Autodesk Inventor part; units mm, degrees
ref_plane "YZ Plane" through (0, 0, 0) normal (1, 0, 0) x (0, 1, 0)
ref_plane "XZ Plane" through (0, 0, 0) normal (0, 1, 0) x (-1, 0, 0)
ref_plane "XY Plane" through (0, 0, 0) normal (0, 0, 1) x (1, 0, 0)
sketch "Sketch1" plane through (0, 0, 0) normal (0, 0, 1) x (1, 0, 0)
  line L0 (-155, -110) -> (155, -110)
  line L1 (155, -110) -> (155, 110)
  line L2 (155, 110) -> (-155, 110)
  line L3 (-155, 110) -> (-155, -110)
  line L4 (-155, -110) -> (155, 110) construction
  line L5 (155, -110) -> (-155, 110) construction
  line L6 (-125, 105) -> (125, 105)
  line L7 (125, 105) -> (125, 99.9)
  line L8 (125, 99.9) -> (-125, 99.9)
  line L9 (-125, 99.9) -> (-125, 105)
  line L10 (150, 80) -> (144.9, 80)
  line L11 (144.9, 80) -> (144.9, -80)
  line L12 (144.9, -80) -> (150, -80)
  line L13 (150, -80) -> (150, 80)
  line L14 (-155, 0) -> (155, 0)
  line L15 (0, 110) -> (0, -110)
  line L16 (-125, -105) -> (125, -105)
  line L17 (125, -105) -> (125, -99.9)
  line L18 (125, -99.9) -> (-125, -99.9)
  line L19 (-125, -99.9) -> (-125, -105)
  line L20 (-150, 80) -> (-144.9, 80)
  line L21 (-144.9, 80) -> (-144.9, -80)
  line L22 (-144.9, -80) -> (-150, -80)
  line L23 (-150, -80) -> (-150, 80)
  point P0 (0, 0)
  point P1 (0, 105)
  point P2 (144.9, 0)
  point P3 (0, -105)
  point P4 (-144.9, 0)
  dimension "d0" = 310
  dimension "d1" = 220
  dimension "d2" = 5.1
  dimension "d3" = 5.1
  dimension "d4" = 30
  dimension "d5" = 30
  dimension "d6" = 5
  dimension "d7" = 5
extrude "Plate1" add sketch "Sketch1" along normal blind 5 contours L3 L14 L23 L22 L21 L15 L18 L19 L16 L0 | L15 L16 L17 L18 L14 L11 L12 L13 L1 L0 | L3 L2 L15 L6 L9 L8 L14 L21 L20 L23 | L14 L13 L10 L11 L15 L8 L7 L6 L2 L1
sketch "Sketch2" plane through (0, 0, 5) normal (0, 0, 1) x (1, 0, 0)
  line L0 (-50, 260) -> (50, 260)
  line L1 (50, 260) -> (50, 110)
  line L2 (50, 110) -> (-50, 110)
  line L3 (-50, 110) -> (-50, 260)
  line L4 (-155, 110) -> (155, 110)
  point P0 (0, 0)
  point P1 (0, 260)
  point P2 (0, 110)
  point P3 (0, 110)
  dimension "d9" = 100
  dimension "d10" = 150
sheet face with bend "Face2" sketch "Sketch2" thickness 5 toward (0, 0, -1) bend radius 5
bend "Bend1"
sketch "Sketch3" plane through (0, 0, 5) normal (0, 0, 1) x (1, 0, 0)
  line L0 (-20, 250.8) -> (20, 250.8)
  line L1 (20, 250.8) -> (20, 256)
  line L2 (20, 256) -> (-20, 256)
  line L3 (-20, 256) -> (-20, 250.8)
  line L4 (-20, 250.8) -> (20, 256) construction
  line L5 (20, 250.8) -> (-20, 256) construction
  line L6 (50, 260) -> (-50, 260)
  line L7 (-46, 155) -> (-40.8, 155)
  line L8 (-40.8, 155) -> (-40.8, 215)
  line L9 (-40.8, 215) -> (-46, 215)
  line L10 (-46, 215) -> (-46, 155)
  line L11 (-46, 155) -> (-40.8, 215) construction
  line L12 (-40.8, 155) -> (-46, 215) construction
  line L13 (-50, 260) -> (-50, 110)
  line L14 (-125, 105) -> (125, 105)
  line L15 (0, 105) -> (0, 260)
  line L16 (46, 155) -> (40.8, 155)
  line L17 (40.8, 155) -> (40.8, 215)
  line L18 (40.8, 215) -> (46, 215)
  line L19 (46, 215) -> (46, 155)
  line L20 (46, 155) -> (40.8, 215) construction
  line L21 (40.8, 155) -> (46, 215) construction
  point P0 (0, 0)
  point P1 (0, 253.4)
  point P2 (-43.4, 185)
  point P3 (-50, 185)
  point P4 (43.4, 185)
  dimension "d16" = 5.2
  dimension "d17" = 4
  dimension "d18" = 40
  dimension "d19" = 5.2
  dimension "d20" = 60
  dimension "d21" = 4
extrude "Cut1" cut sketch "Sketch3" against normal blind 5
feature "Corner Round1" [suppressed]
equation "\"d7\" = d6"
equation "\"d21\" = d17"
equation "\"d22\" = Thickness"
equation "\"d8\" = Thickness"
equation "\"d11\" = BendRadius"
equation "\"d12\" = BendReliefWidth"
equation "\"d14\" = MinimumRemnant"
equation "\"d13\" = BendReliefDepth"
equation "\"d15\" = TransitionRadius"
equation "\"BendRadius\" = Thickness"
equation "\"BendReliefWidth\" = Thickness"
equation "\"BendReliefDepth\" = 0.5 * Thickness"
equation "\"TransitionRadius\" = BendRadius"
equation "\"JacobiRadiusSize\" = BendRadius"
equation "\"GapSize\" = Thickness"
properties part number "Finishing Sheets .5 ( Buttom )"
Work out the finished part from the listing and answer in its coordinate system (mm). Give positions to 0.01 mm unless a question says otherwise; leave off trailing zeros. Loops run counter-clockwise (first coordinate to the right, second up) from the corner with the lowest first, then second, coordinate; pieces in that order, holes last. Notation, with made-up numbers: (14.5, 82.25) -> (18.5, 82.25) arc R17 cw to (18.5, 103.25) -> close; hole circle Ø6 at (30.25, 72.25). An arc over 180 degrees is marked (long way). Use a Markdown table: item, result. Add a question column.
1. Section B-B on x = -65.5 is taken. Determine the outline of the cut face in (y, z), and give its area (3 significant figures).
2. Find the intervals of material crossed by probe 1 along X at (y, z) = (182, 2.55); probe 2 along Y at (x, z) = (54.5, 4.1); probe 3 along X at (y, z) = (-52.5, 1.1), in increasing order.
3. Section C-C on y = 30.5 is taken. Determine the outline of the cut face in (x, z).
4. Section D-D on z = 3.75 is taken. State how many separate pieces and enclosed holes the cut face has, and give its area (3 significant figures).
5. Flat-ended cylindrical pins translate along their axes: pin 1 Ø2 at (x, z) = (-108.5, 2) entering from +Y; pin 2 Ø1.5 at (y, z) = (187, 2.5) entering from +X. Find the tip coordinate at first contact, or state that the pin passes through.
6. Section A-A on x = -7.5 is taken. Determine the outline of the cut face in (y, z).
Results below:
| question | item | result |
|---|---|---|
| 1 | outline | (-110, 0) -> (-105, 0) -> (-105, 5) -> (-110, 5) -> close; (-99.9, 0) -> (99.9, 0) -> (99.9, 5) -> (-99.9, 5) -> close; (105, 0) -> (110, 0) -> (110, 5) -> (105, 5) -> close |
| 1 | area | 1,050 mm^2 |
| 2 | probe 1 | x = -50 to -46, -40.8 to 40.8, 46 to 50 |
| 2 | probe 2 | y = -110 to -105, -99.9 to 99.9, 105 to 110 |
| 2 | probe 3 | x = -155 to -150, -144.9 to 144.9, 150 to 155 |
| 3 | outline | (-155, 0) -> (-150, 0) -> (-150, 5) -> (-155, 5) -> close; (-144.9, 0) -> (144.9, 0) -> (144.9, 5) -> (-144.9, 5) -> close; (150, 0) -> (155, 0) -> (155, 5) -> (150, 5) -> close |
| 4 | separate pieces | 1 |
| 4 | enclosed holes | 7 |
| 4 | area | 78,200 mm^2 |
| 5 | pin 1 | stops at y = 110 |
| 5 | pin 2 | stops at x = 50 |
| 6 | outline | (-110, 0) -> (-105, 0) -> (-105, 5) -> (-110, 5) -> close; (-99.9, 0) -> (99.9, 0) -> (99.9, 5) -> (-99.9, 5) -> close; (105, 0) -> (250.8, 0) -> (250.8, 5) -> (105, 5) -> close; (256, 0) -> (260, 0) -> (260, 5) -> (256, 5) -> close |
